Design review of the part shown in the three views and the two pictorial views. Dimensions are in mm from the part's minimum x, y and z. A direction names the side the tool comes from. Coordinates: 2 decimals unless noted, no trailing zeros. Write each loop counter-clockwise with the first axis right and the second up, starting at its lowest first coordinate (ties: lowest second). Pieces come first, ordered by that corner, then holes. Notation, with made-up numbers: (69, -4.5) -> (103, -4.5) arc R19 cw to (103, 25.5) -> close; hole circle Ø6 at (69.25, -38.5). An arc over 180 degrees is marked (long way). Answer in a Markdown table with one row per item. Add a question column.
Item 1: Take a section at B-B, the plane y = 37. Write out the cut boundary in (x, z), and give its area (3 significant figures).
Item 2: For the marked faces 1 and 2, list the 3-axis set-ups (+Z, -Z, +X, -X, +Y, -Y) from which the entire face can be reached by the end or side of a thin tool; tool diameter is ignored.
Item 3: Clearance check with flat-ended pins moving along their axes: P1, Ø3, axis at y = 14, z = 9, coming from the -X side; P2, Ø1, axis at y = 68.5, z = 8, coming from the +X side; P3, Ø2, axis at x = 6.5, y = 31.5, coming from the +Z side; P4, Ø5, axis at x = 6, z = 7.5, coming from the -Y side. State where each tip first meets the part, or that it passes through.
Item 4: Take a section at A-A, the plane x = 5.8. Write out the cut boundary in (y, z).
Item 5: To check wall thickness, follow line 1 (Y direction, x = 3.75, z = 8.25); line 2 (X direction, y = 11, z = 5.5); line 3 (X direction, y = 72, z = 4). State the ranges of each line that lie inside material, in increasing order.
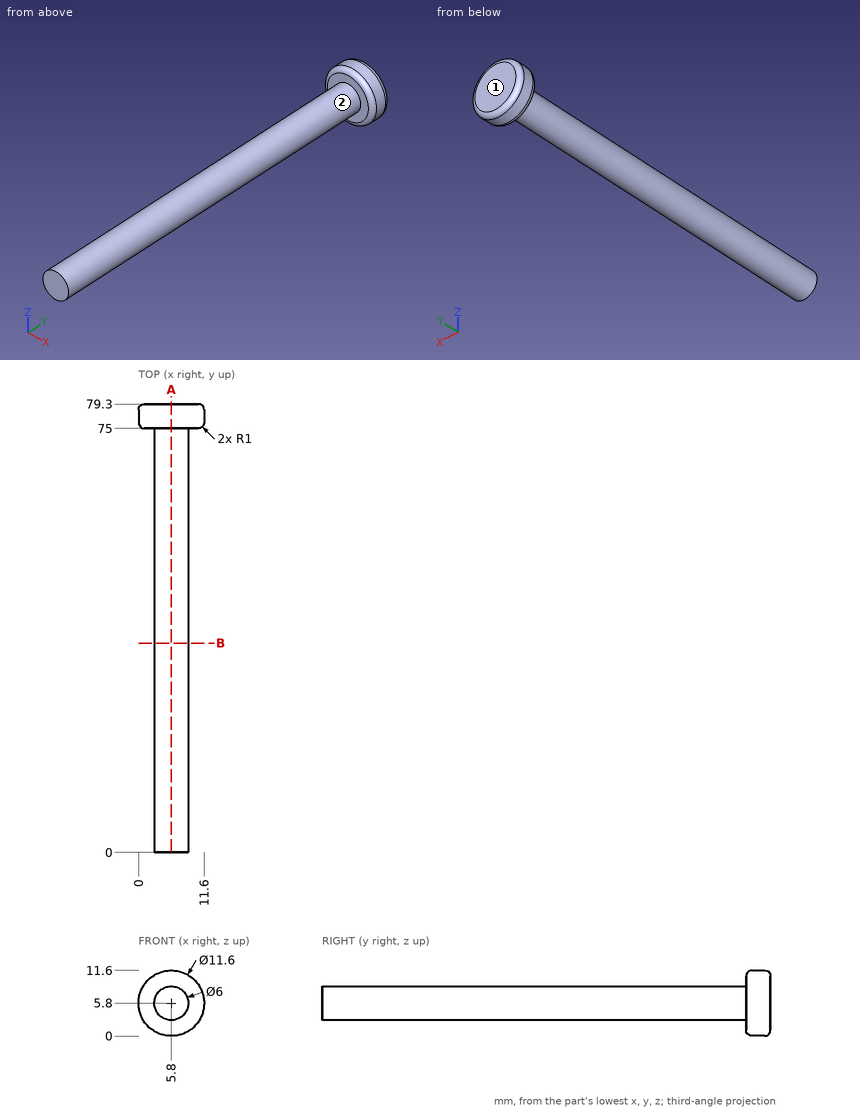
Answers:
| question | item | result |
|---|---|---|
| 1 | outline | circle Ø6 at (5.8, 5.8) |
| 1 | area | 28.3 mm^2 |
| 2 | face 1 | +Z, -Z, +X, -X, +Y |
| 2 | face 2 | -Y |
| 3 | P1 | stops at x = 3.33 |
| 3 | P2 | stops at x = 8.27 |
| 3 | P3 | stops at z = 8.8 |
| 3 | P4 | stops at y = 0 |
| 4 | outline | (0, 2.8) -> (75, 2.8) -> (75, 1) arc R1 ccw to (76, 0) -> (78.3, 0) arc R1 ccw to (79.3, 1) -> (79.3, 10.6) arc R1 ccw to (78.3, 11.6) -> (76, 11.6) arc R1 ccw to (75, 10.6) -> (75, 8.8) -> (0, 8.8) -> close |
| 5 | line 1 | y = 75 to 79.3 |
| 5 | line 2 | x = 2.82 to 8.78 |
| 5 | line 3 | x = 3.4 to 8.2 |
